```python
from build123d import *

# Parameters (mm, degrees)
EXTRUDE1_DEPTH = 533.4


with BuildPart() as part:
    # Sketch1 → Extrude1 (new body, symmetric)
    with BuildSketch(Plane.XY):
        with BuildLine():
            Line((1169.5811, 22.86), (1169.5811, 18.542))
            Line((1169.5811, 18.542), (1167.2189, 18.542))
            Line((1167.2189, 18.542), (1167.2189, 22.86))
            Line((1167.2189, 22.86), (1160.272, 22.86))
            Line((1160.272, 22.86), (1160.272, 24.13))
            Line((1160.272, 24.13), (1167.2189, 24.13))
            Line((1167.2189, 24.13), (1167.2189, 30.988))
            ThreePointArc((1167.2189, 30.988), (1163.937883426, 30.530285143), (1160.907403243, 29.192091395))
            Line((1160.907403243, 29.192091395), (1160.483801081, 30.389363798))
            ThreePointArc((1160.483801081, 30.389363798), (1164.93748479, 31.786014706), (1169.5811, 32.258))
            Line((1169.5811, 32.258), (1169.5811, 24.13))
            Line((1169.5811, 24.13), (1176.528, 24.13))
            Line((1176.528, 24.13), (1176.528, 22.86))
            Line((1176.528, 22.86), (1169.5811, 22.86))
        make_face()
    extrude(amount=EXTRUDE1_DEPTH, both=True)


solid = part.part
```
Check sheet for the modelled part. Datum: model origin and axes. Units: mm. Round coordinates to 2 decimals unless told otherwise and drop trailing zeros. Order: outer loops, then holes, each group sorted by start corner. A loop starts at its lowest first (then second) coordinate and runs counter-clockwise, first axis right, second up. Notation, with made-up numbers: (-8.75, -9) -> (27.25, -9) arc R10 cw to (27.25, 10) -> close; hole circle Ø11 at (-11, 66.25). An arc over 180 degrees is marked (long way). Use CSV: the item, a comma, the result in double quotes.
(1) Material ranges on line 1 along X through (y, z) = (26.5, -128.5); line 2 along Y through (x, z) = (1166, 30); line 3 along X through (y, z) = (30, -25), recorded low to high. Write a range as from..to.
Worked out:
line 1,"1167.22..1169.58"
line 2,"22.86..24.13, 30.93..31.98"
line 3,"1160.62..1162.45, 1167.22..1169.58"
(2) Cross-section at B-B (x = 1163.75). Record the boundary of the cut face in (y, z).
Worked out:
outline,"(22.86, -533.4) -> (24.13, -533.4) -> (24.13, 533.4) -> (22.86, 533.4) -> close; (30.48, -533.4) -> (31.51, -533.4) -> (31.51, 533.4) -> (30.48, 533.4) -> close"
(3) Cross-section at A-A (z = 132.5). Record the boundary of the cut face in (x, y).
Worked out:
outline,"(1160.27, 22.86) -> (1167.22, 22.86) -> (1167.22, 18.54) -> (1169.58, 18.54) -> (1169.58, 22.86) -> (1176.53, 22.86) -> (1176.53, 24.13) -> (1169.58, 24.13) -> (1169.58, 32.26) arc R23.08 ccw to (1160.48, 30.39) -> (1160.91, 29.19) arc R11.99 cw to (1167.22, 30.99) -> (1167.22, 24.13) -> (1160.27, 24.13) -> close"
(4) Depth check by flat-ended pin: pin 1 (4.5 mm diameter, centred on y = 20.5, z = 50.5, fed in from +X); pin 2 (1 mm diameter, centred on x = 1167, y = 26, fed in from -Z); pin 3 (1 mm diameter, centred on x = 1170.5, z = 415.5, fed in from -Y); pin 4 (7.5 mm diameter, centred on y = 28, z = 94.5, fed in from -X). Enter the tip coordinate at first touch or a pass-through.
Worked out:
pin 1,"x = 1169.58"
pin 2,"z = -533.4"
pin 3,"y = 22.86"
pin 4,"x = 1160.48"
